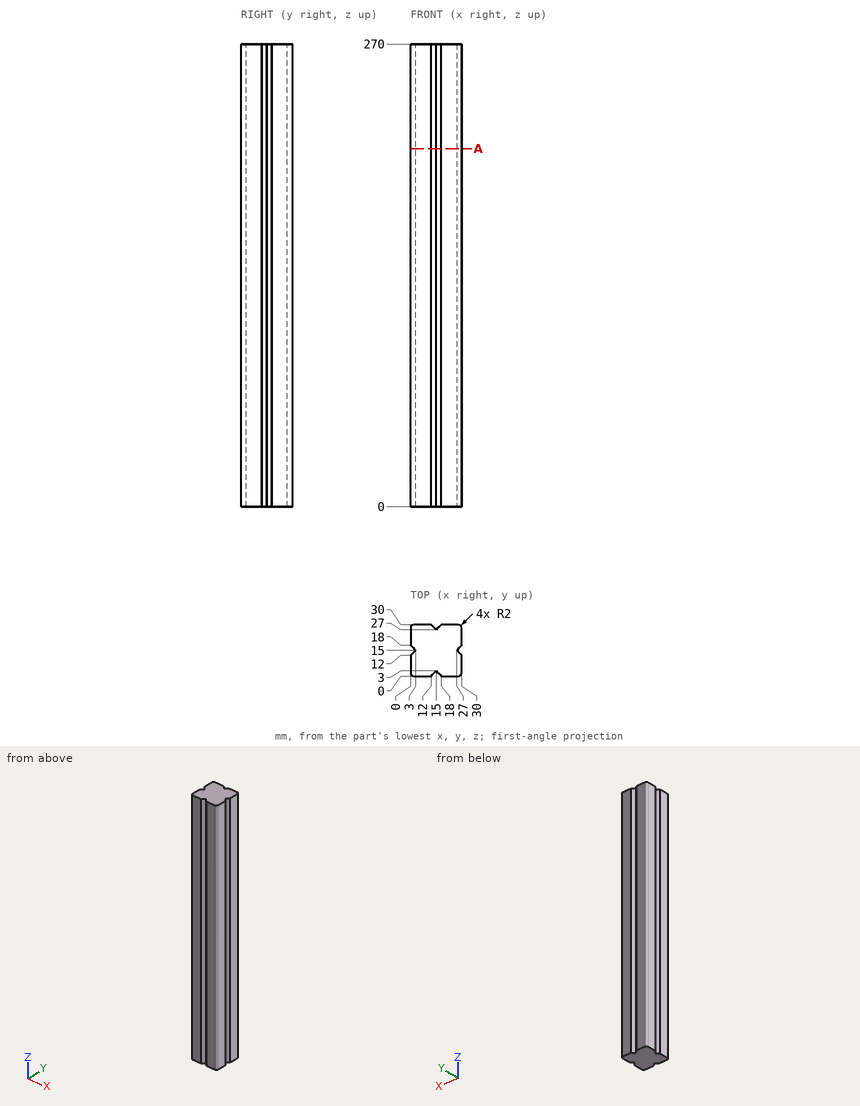
Geometry check sheet. Reference: drawing and pictorial views, mm from the part's lowest x, y, z. Give positions to 0.01 mm unless a question says otherwise; leave off trailing zeros. Order: outer loops, then holes, each group sorted by start corner. A loop starts at its lowest first (then second) coordinate and runs counter-clockwise, first axis right, second up. Notation, with made-up numbers: (61.25, 5) -> (100.25, 5) arc R31 cw to (100.25, 41) -> close; hole circle Ø6 at (49.25, 34.5). An arc over 180 degrees is marked (long way). Write each question's results on one line, items separated by ' | '. Start each with the question number.
(1) Sectioned sample at A-A (z = 209). Enter the section's corners in (x, y), plus the area to 3 significant figures.
(2) Scan lines: line 1 (Y direction, x = 2.75, z = 110); line 2 (Y direction, x = 2, z = 22.5). Record each from-to range of solid material in increasing order.
(3) Gauge pin test, flat end, axial feed: P1, Ø1.5, axis at y = 16, z = 193, coming from the -X side. Record the tip position at first contact, or that the pin passes through.
Answer below:
1) outline: (0, 2) arc R2 ccw to (2, 0) -> (12, 0) -> (15, 3) -> (18, 0) -> (28, 0) arc R2 ccw to (30, 2) -> (30, 12) -> (27, 15) -> (30, 18) -> (30, 28) arc R2 ccw to (28, 30) -> (18, 30) -> (15, 27) -> (12, 30) -> (2, 30) arc R2 ccw to (0, 28) -> (0, 18) -> (3, 15) -> (0, 12) -> close | area: 861 mm2
2) line 1: 0 to 14.75, 15.25 to 30 | line 2: 0 to 14, 16 to 30
3) P1: x = 1.25
